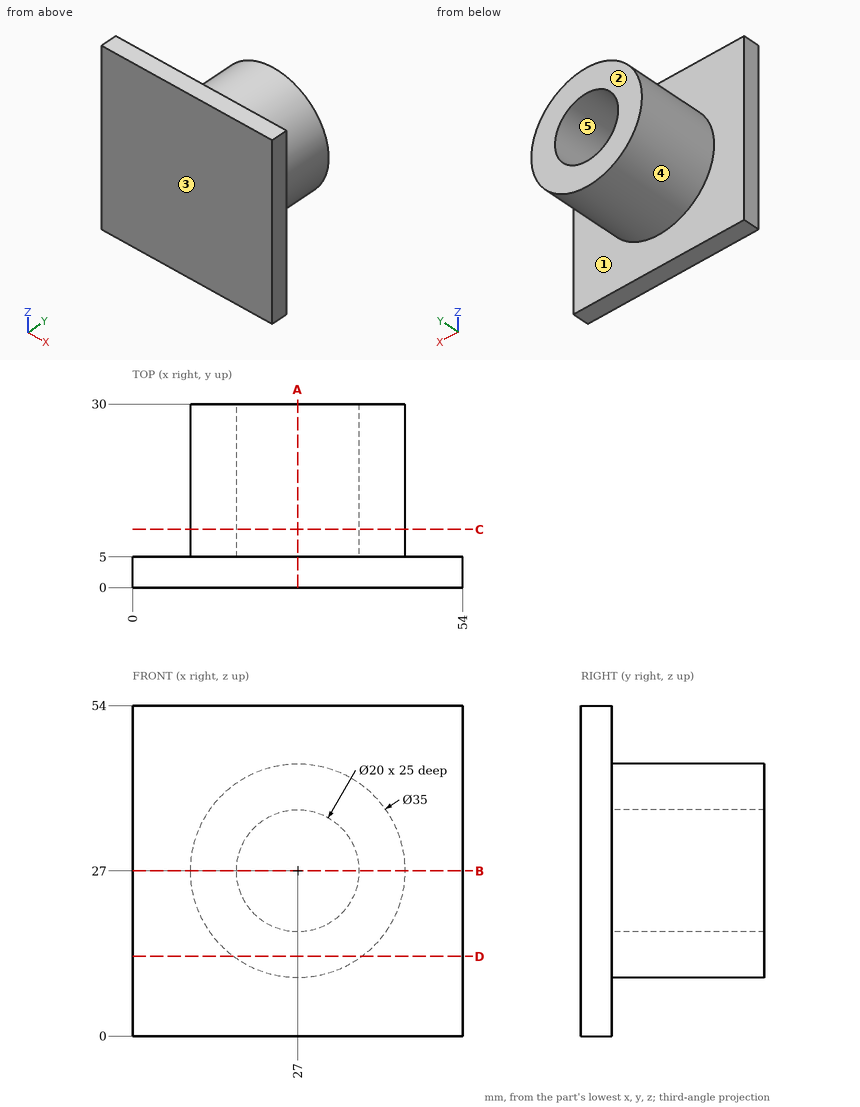
Source: three-view drawing plus pictorial views. Frame: mm from the lowest corner of the part. A direction names the side the tool comes from. Round coordinates to 2 decimals unless told otherwise and drop trailing zeros. Order: outer loops, then holes, each group sorted by start corner. A loop starts at its lowest first (then second) coordinate and runs counter-clockwise, first axis right, second up. Notation, with made-up numbers: (63.25, 81) -> (114.25, 81) arc R32 ccw to (114.25, 108) -> close; hole circle Ø1 at (-21, 42). An arc over 180 degrees is marked (long way). Use one line per item in the form item = value. Start each with the question number.
1. Pin query (flat end, axial travel): pin 1 Ø10 at (x, z) = (23, 26.5) entering from +Y; pin 2 Ø12 at (x, y) = (30.5, 20) entering from -Z; pin 3 Ø1.5 at (y, z) = (17.5, 19) entering from +X. Return the tip coordinate at first contact, or that it passes through.
2. Cut plane B-B (z = 27). Return the cut outline in (x, y), then the cut area to 3 significant figures.
3. Cut plane A-A (x = 27). Return the cut outline in (y, z), then the cut area to 3 significant figures.
4. Cut plane D-D (z = 13). Return the cut outline in (x, y).
5. Reachability of the marked faces 1 and 2 from +Z, -Z, +X, -X, +Y, -Y: full face, straight path, thin tool, end or side. Return the list, or none.
6. Line query: probe 1 along X at (y, z) = (20.75, 27.5); probe 2 along Z at (x, y) = (27, 24); probe 3 along Y at (x, z) = (41.5, 7.5). Output: solid intervals per line, ascending.
7. Cut plane C-C (y = 9.5). Return the cut outline in (x, z), then the cut area to 3 significant figures.
8. Draft query along X for the marked faces 3, 4 and 5. Return one class per face: pulls with the +X half, pulls with the -X half, needs draft (parallel to the pull), parting line crosses it, or undercut.
Solution:
q1.pin_1 = 5
q1.pin_2 = 9.5
q1.pin_3 = 42.93
q2.outline = (0, 0) -> (54, 0) -> (54, 5) -> (44.5, 5) -> (44.5, 30) -> (37, 30) -> (37, 5) -> (17, 5) -> (17, 30) -> (9.5, 30) -> (9.5, 5) -> (0, 5) -> close
q2.area = 645 mm^2
q3.outline = (0, 0) -> (5, 0) -> (5, 9.5) -> (30, 9.5) -> (30, 17) -> (5, 17) -> (5, 37) -> (30, 37) -> (30, 44.5) -> (5, 44.5) -> (5, 54) -> (0, 54) -> close
q3.area = 645 mm^2
q4.outline = (0, 0) -> (54, 0) -> (54, 5) -> (37.5, 5) -> (37.5, 30) -> (16.5, 30) -> (16.5, 5) -> (0, 5) -> close
q5.face_1 = +Y
q5.face_2 = +Z, -Z, +X, -X, +Y
q6.probe_1 = 9.51 to 17.01, 36.99 to 44.49
q6.probe_2 = 9.5 to 17, 37 to 44.5
q6.probe_3 = 0 to 5
q7.outline = circle Ø35 at (27, 27); hole circle Ø20 at (27, 27)
q7.area = 648 mm^2
q8.face_3 = needs draft
q8.face_4 = parting line crosses it
q8.face_5 = undercut
